Design review of the part built by this model. Coordinates are the model's own, in mm. Face numbers are marked on the shaded views. A direction names the side the tool comes from. Coordinates: 2 decimals unless noted, no trailing zeros.
Q1. For pin 1 Ø12 at (x, y) = (-15.5, -10.5) entering from +Z; pin 2 Ø8 at (y, z) = (17.5, -6.5) entering from +X; pin 3 Ø8 at (x, z) = (-12.5, 5) entering from +Y, all flat-tipped, find the tip position at first contact; note any pin that passes through.
Q2. The part is to be moulded in two halves that separate along Y. For the marked faces 3 and 4, say which applies: released by +Y, released by -Y, zero draft, split by the parting line, or undercut.
Q3. Take a section at A-A, the plane z = 2.5. State how many separate pieces and enclosed holes the cut face has, plus the area to 3 significant figures.
Q4. For the marked faces 1 and 2, list the 3-axis set-ups (+Z, -Z, +X, -X, +Y, -Y) from which the entire face can be reached by the end or side of a thin tool; tool diameter is ignored.
Q5. For L1, parallel to X at y = -9.5, z = -3.5; L2, parallel to Y at x = 4, z = 4; L3, parallel to Y at x = 4.5, z = -7, list the stretches that pass through material, from the lowest coordinate up.
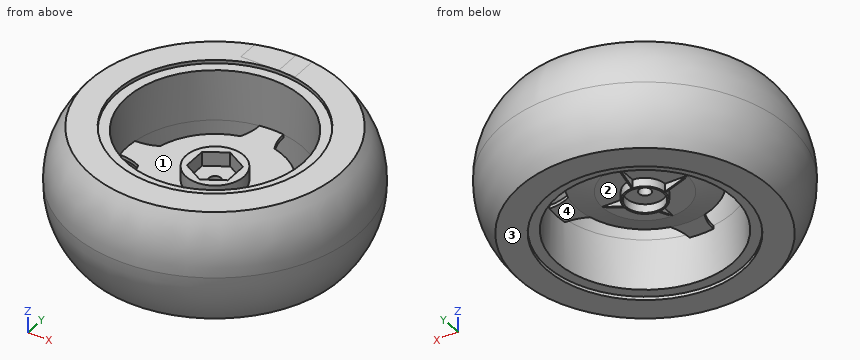
from build123d import *
from build123d.topology import SkipClean

# Parameters (mm, degrees)
SKETCH2_R            = 20
BOSS_EXTRUDE1_DEPTH  = 1
SKETCH3_R            = 8.5
BOSS_EXTRUDE2_DEPTH  = 4.2
BOSS_EXTRUDE4_DEPTH  = 2.5
BOSS_EXTRUDE5_DEPTH  = 3.5
CUT_EXTRUDE1_DEPTH   = 2.5
SKETCH14_R           = 1.75
CUT_EXTRUDE2_DEPTH   = 20.5
BOSS_EXTRUDE7_DEPTH  = 2.56
BOSS_EXTRUDE8_DEPTH  = 2.56
CUT_EXTRUDE4_DEPTH   = 1
CIRPATTERN3_COUNT    = 4
BOSS_EXTRUDE10_DEPTH = 2.56
SKETCH22_R           = 29
SKETCH22_R_2         = 26
BOSS_EXTRUDE11_DEPTH = 15
BOSS_EXTRUDE12_START = 15
SKETCH23_R           = 29
SKETCH23_R_2         = 26
BOSS_EXTRUDE12_DEPTH = 15
SKETCH25_R           = 37
SKETCH25_R_2         = 29
BOSS_EXTRUDE14_DEPTH = 16
BOSS_EXTRUDE15_START = 16
SKETCH26_R           = 37
SKETCH26_R_2         = 29
BOSS_EXTRUDE15_DEPTH = 16
SKETCH27_W           = 4.936524623
SKETCH27_H           = 8
BOSS_EXTRUDE16_DEPTH = 16
SKETCH29_W           = 16
SKETCH29_H           = 8
CUT_EXTRUDE5_DEPTH   = 16


with BuildPart() as part:
    # Sketch2 → Boss-Extrude1 (new body)
    with BuildSketch(Plane.XY):
        Circle(SKETCH2_R)
    extrude(amount=BOSS_EXTRUDE1_DEPTH)

    # Sketch3 → Boss-Extrude2 (add)
    with BuildSketch(Plane.XY.offset(1)):
        Circle(SKETCH3_R)
        Polygon((0, 6.95), (-6.018876556, 3.475), (-6.018876556, -3.475), (0, -6.95), (6.018876556, -3.475), (6.018876556, 3.475), align=None, mode=Mode.SUBTRACT)
    extrude(amount=BOSS_EXTRUDE2_DEPTH)

    # Sketch7 → Boss-Extrude4 (add)
    with BuildSketch(Plane(origin=(0, 0, 0), x_dir=(-1, 0, 0), z_dir=(0, 0, -1))):
        with BuildLine():
            Line((-12.53, 0), (0, 0))
            Line((0, 0), (12.53, 0))
            ThreePointArc((12.53, 0), (0, 12.53), (-12.53, 0))
        make_face()
    extrude(amount=BOSS_EXTRUDE4_DEPTH)

    # Sketch10 → Revolve1 (revolve)
    with BuildSketch(Plane.XZ):
        Polygon((12.53, -2.5), (20, 0), (12.53, 0), (0, 0), (0, -2.5), align=None)
    revolve(axis=Axis((0, 0, 0), (0, 0, -1)))

    # Sketch11 → Boss-Extrude5 (add)
    with BuildSketch(Plane(origin=(0, 0, -2.5), x_dir=(-1, 0, 0), z_dir=(0, 0, -1))):
        with BuildLine():
            ThreePointArc((25.763346056, -3.5), (22.477394983, -3.88001547), (19.364916731, -5))
            ThreePointArc((19.364916731, -5), (20, 0), (19.364916731, 5))
            ThreePointArc((19.364916731, 5), (22.477394983, 3.88001547), (25.763346056, 3.5))
            ThreePointArc((25.763346056, 3.5), (26, 0), (25.763346056, -3.5))
        make_face()
        with BuildLine():
            ThreePointArc((3.5, 25.763346056), (3.88001547, 22.477394983), (5, 19.364916731))
            ThreePointArc((5, 19.364916731), (0, 20), (-5, 19.364916731))
            ThreePointArc((-5, 19.364916731), (-3.88001547, 22.477394983), (-3.5, 25.763346056))
            ThreePointArc((-3.5, 25.763346056), (0, 26), (3.5, 25.763346056))
        make_face()
        with BuildLine():
            ThreePointArc((-3.5, -25.763346056), (-3.88001547, -22.477394983), (-5, -19.364916731))
            ThreePointArc((-5, -19.364916731), (0, -20), (5, -19.364916731))
            ThreePointArc((5, -19.364916731), (3.88001547, -22.477394983), (3.5, -25.763346056))
            ThreePointArc((3.5, -25.763346056), (0, -26), (-3.5, -25.763346056))
        make_face()
        with BuildLine():
            ThreePointArc((-25.763346056, 3.5), (-22.477394983, 3.88001547), (-19.364916731, 5))
            ThreePointArc((-19.364916731, 5), (-20, 0), (-19.364916731, -5))
            ThreePointArc((-19.364916731, -5), (-22.477394983, -3.88001547), (-25.763346056, -3.5))
            ThreePointArc((-25.763346056, -3.5), (-26, 0), (-25.763346056, 3.5))
        make_face()
    extrude(amount=-BOSS_EXTRUDE5_DEPTH)

    # Sketch13 → Cut-Extrude1 (cut)
    with BuildSketch(Plane(origin=(0, 0, -2.5), x_dir=(-1, 0, 0), z_dir=(0, 0, -1))):
        with BuildLine():
            ThreePointArc((-3.5, -25.763346056), (0, -26), (3.5, -25.763346056))
            ThreePointArc((3.5, -25.763346056), (3.88001547, -22.477394983), (5, -19.364916731))
            ThreePointArc((5, -19.364916731), (0, -20), (-5, -19.364916731))
            ThreePointArc((-5, -19.364916731), (-3.88001547, -22.477394983), (-3.5, -25.763346056))
        make_face()
        with BuildLine():
            ThreePointArc((5, 19.364916731), (0, 20), (-5, 19.364916731))
            ThreePointArc((-5, 19.364916731), (-3.88001547, 22.477394983), (-3.5, 25.763346056))
            ThreePointArc((-3.5, 25.763346056), (0, 26), (3.5, 25.763346056))
            ThreePointArc((3.5, 25.763346056), (3.88001547, 22.477394983), (5, 19.364916731))
        make_face()
        with BuildLine():
            ThreePointArc((25.763346056, -3.5), (22.477394983, -3.88001547), (19.364916731, -5))
            ThreePointArc((19.364916731, -5), (20, 0), (19.364916731, 5))
            ThreePointArc((19.364916731, 5), (22.477394983, 3.88001547), (25.763346056, 3.5))
            ThreePointArc((25.763346056, 3.5), (26, 0), (25.763346056, -3.5))
        make_face()
        with BuildLine():
            ThreePointArc((-25.763346056, -3.5), (-22.477394983, -3.88001547), (-19.364916731, -5))
            ThreePointArc((-19.364916731, -5), (-20, 0), (-19.364916731, 5))
            ThreePointArc((-19.364916731, 5), (-22.477394983, 3.88001547), (-25.763346056, 3.5))
            ThreePointArc((-25.763346056, 3.5), (-26, 0), (-25.763346056, -3.5))
        make_face()
    extrude(amount=-CUT_EXTRUDE1_DEPTH, mode=Mode.SUBTRACT)

    # Sketch14 → Cut-Extrude2 (cut)
    with BuildSketch(Plane(origin=(0, 0, -2.5), x_dir=(-1, 0, 0), z_dir=(0, 0, -1))):
        Circle(SKETCH14_R)
    extrude(amount=-CUT_EXTRUDE2_DEPTH, mode=Mode.SUBTRACT)

    # Sketch15 → Boss-Extrude7 (add)
    with BuildSketch(Plane(origin=(0, 0, -2.5), x_dir=(-1, 0, 0), z_dir=(0, 0, -1))):
        with BuildLine():
            ThreePointArc((-5.5, 0), (0, 5.5), (5.5, 0))
            Line((5.5, 0), (6, 0))
            ThreePointArc((6, 0), (0, 6), (-6, 0))
            Line((-6, 0), (-5.5, 0))
        make_face()
    extrude(amount=BOSS_EXTRUDE7_DEPTH)

    # Sketch18 → Boss-Extrude8 (add)
    with BuildSketch(Plane(origin=(0, 0, -2.5), x_dir=(-1, 0, 0), z_dir=(0, 0, -1))):
        with BuildLine():
            Line((12.528403729, 0.2), (5.99666574, 0.2))
            ThreePointArc((5.99666574, 0.2), (6, 0), (5.99666574, -0.2))
            Line((5.99666574, -0.2), (12.528403729, -0.2))
            ThreePointArc((12.528403729, -0.2), (12.53, 0), (12.528403729, 0.2))
        make_face()
    boss_extrude8 = extrude(amount=BOSS_EXTRUDE8_DEPTH)

    # Sketch19 → Cut-Extrude4 (cut)
    with BuildSketch(Plane.XZ.offset(0.2)):
        Polygon((-12.528403729, -5.06), (-13.38680772, -5.06), (-13.38680772, -2.5), (-12.528403729, -2.5), (-5.99666574, -4.849997635), (-5.99666574, -5.06), align=None)
    cut_extrude4 = extrude(amount=-CUT_EXTRUDE4_DEPTH, mode=Mode.SUBTRACT)

    # CirPattern3: Boss-Extrude8, Cut-Extrude4 ×4 about axis
    cirpattern3_axis = Axis((0, 0, 0), (0, 0, 1))
    add([boss_extrude8.rotate(cirpattern3_axis, i * 360 / CIRPATTERN3_COUNT) for i in range(1, CIRPATTERN3_COUNT)])
    add([cut_extrude4.rotate(cirpattern3_axis, i * 360 / CIRPATTERN3_COUNT) for i in range(1, CIRPATTERN3_COUNT)], mode=Mode.SUBTRACT)

    # Sketch20 → Boss-Extrude10 (add)
    with SkipClean():  # the faces are left unmerged after this step: merging them gives an invalid solid
        with BuildSketch(Plane(origin=(0, 0, -2.5), x_dir=(-1, 0, 0), z_dir=(0, 0, -1))):
            with BuildLine():
                Line((-6, 0), (-5.5, 0))
                ThreePointArc((-5.5, 0), (0, -5.5), (5.5, 0))
                Line((5.5, 0), (6, 0))
                ThreePointArc((6, 0), (0, -6), (-6, 0))
            make_face()
        extrude(amount=BOSS_EXTRUDE10_DEPTH)



with BuildPart() as body_2:
    # Sketch22 → Boss-Extrude11 (new body)
    with BuildSketch(Plane.XY.offset(1)):
        Circle(SKETCH22_R)
        Circle(SKETCH22_R_2, mode=Mode.SUBTRACT)
    extrude(amount=BOSS_EXTRUDE11_DEPTH)


with BuildPart() as part_1:
    with SkipClean():  # the faces are left unmerged after this step: merging them gives an invalid solid
        add(part.part)

        add(body_2.part)  # Boss-Extrude12 merges body 2
        # Sketch23 → Boss-Extrude12 (add)
        with BuildSketch(Plane(origin=(0, 0, 1), x_dir=(-1, 0, 0), z_dir=(0, 0, -1)).offset(BOSS_EXTRUDE12_START)):
            with Locations(Location((0, 0, 0), (0, 0, 180))):
                Circle(SKETCH23_R)
            with Locations(Location((0, 0, 0), (0, 0, 180))):
                Circle(SKETCH23_R_2, mode=Mode.SUBTRACT)
        extrude(amount=-BOSS_EXTRUDE12_DEPTH)

    # Sketch25 → Boss-Extrude14 (add)
    with SkipClean():  # the faces are left unmerged after this step: merging them gives an invalid solid
        with BuildSketch(Plane.XY.offset(1)):
            Circle(SKETCH25_R)
            Circle(SKETCH25_R_2, mode=Mode.SUBTRACT)
        extrude(amount=BOSS_EXTRUDE14_DEPTH)

    # Sketch26 → Boss-Extrude15 (add)
    with SkipClean():  # the faces are left unmerged after this step: merging them gives an invalid solid
        with BuildSketch(Plane(origin=(0, 0, 1), x_dir=(-1, 0, 0), z_dir=(0, 0, -1)).offset(BOSS_EXTRUDE15_START)):
            Circle(SKETCH26_R)
            with Locations(Location((0, 0, 0), (0, 0, 180))):
                Circle(SKETCH26_R_2, mode=Mode.SUBTRACT)
        extrude(amount=-BOSS_EXTRUDE15_DEPTH)

    # Sketch27 → Boss-Extrude16 (add)
    with SkipClean():  # the faces are left unmerged after this step: merging them gives an invalid solid
        with BuildSketch(Plane.XY.offset(17)):
            with Locations((2.468262312, 33)):
                Rectangle(SKETCH27_W, SKETCH27_H)
        extrude(amount=BOSS_EXTRUDE16_DEPTH)

    # Sketch28 → Revolve2 (revolve)
    with SkipClean():  # the faces are left unmerged after this step: merging them gives an invalid solid
        with BuildSketch(Plane.ZY):
            with BuildLine():
                ThreePointArc((1, 42.5), (9.485130196, 41.161287844), (17, 37))
                Line((17, 37), (-15, 37))
                ThreePointArc((-15, 37), (-7.485130196, 41.161287844), (1, 42.5))
            make_face()
        revolve(axis=Axis((0, 0, -15), (0, 0, 1)))

    # Sketch29 → Cut-Extrude5 (cut)
    with SkipClean():  # the faces are left unmerged after this step: merging them gives an invalid solid
        with BuildSketch(Plane(origin=(4.936524623, 0, 0), x_dir=(0, 0, -1), z_dir=(1, 0, 0))):
            with Locations((-25, 33)):
                Rectangle(SKETCH29_W, SKETCH29_H)
        extrude(amount=-CUT_EXTRUDE5_DEPTH, mode=Mode.SUBTRACT)


solid = part_1.part
Responses:
1. pin 1: stops at z = 1
1. pin 2: stops at x = 39.57
1. pin 3: stops at y = 41.5
2. face 3: zero draft
2. face 4: undercut
3. separate pieces: 2
3. enclosed holes: 2
3. area: 3,650 mm2
4. face 1: +Z
4. face 2: -Z
5. L1: x = -41.09 to -24.2, -0.2 to 0.2, 24.2 to 41.09
5. L2: y = -42.18 to -25.69, -7.5 to -4.64, 4.64 to 7.5, 25.69 to 42.18
5. L3: y = -41.08 to -25.61, 25.61 to 41.08
